Drawing for the job (mm, zero at the part's lowest x, y, z). Round coordinates to 2 decimals unless told otherwise and drop trailing zeros. Write each loop counter-clockwise with the first axis right and the second up, starting at its lowest first coordinate (ties: lowest second). Pieces come first, ordered by that corner, then holes.
Item 1: Band-saw the part on A-A, the plane x = 13.5. Write the cut outline in (y, z).
Item 2: Mould opens along Y. For the marked faces 1, 2, 3 and 4 say: +Y half, -Y half, draft (parallel to the pull), parting line (faces both ways), or undercut.
Item 3: Band-saw the part on D-D, the plane x = 25. Write the cut outline in (y, z), then the cut area to 4 significant figures.
Item 4: Wall check: probe 1 along Y at (x, z) = (13.5, 1.8); probe 2 along X at (y, z) = (14.5, 1.15). Give the ranges that are in metal, low to high.
Item 5: Band-saw the part on C-C, the plane z = 2.65. Count the separate pieces of the cut face and the enclosed holes in it, then the cut area to 3 significant figures.
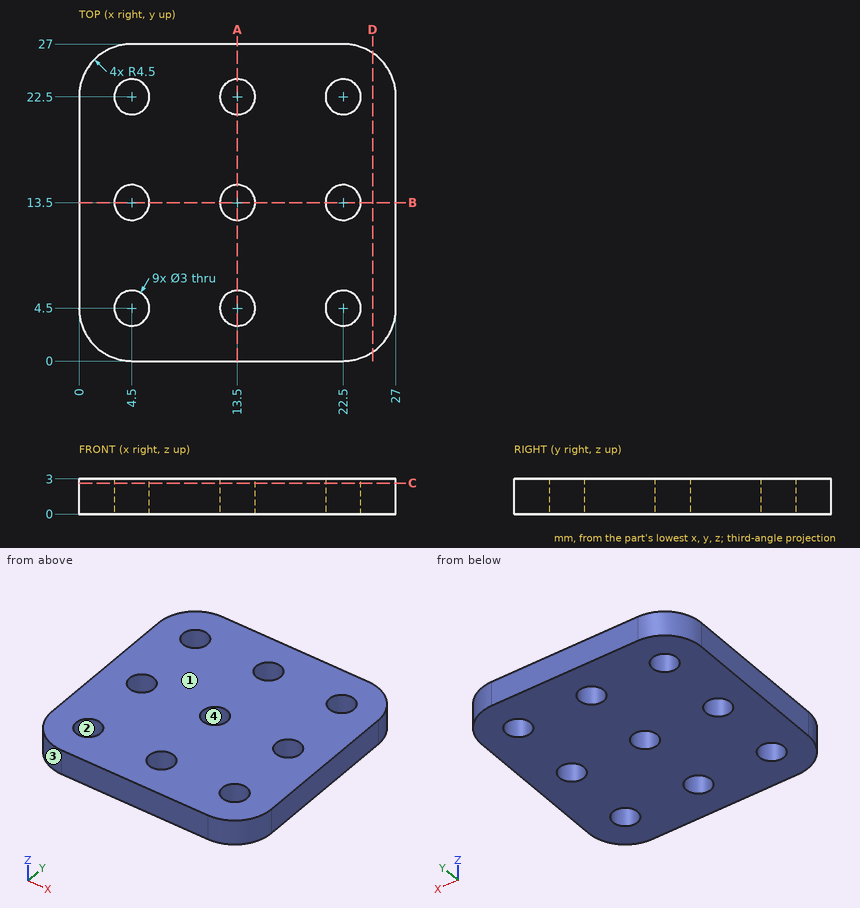
Results:
1. outline: (0, 0) - (3, 0) - (3, 3) - (0, 3) - close; (6, 0) - (12, 0) - (12, 3) - (6, 3) - close; (15, 0) - (21, 0) - (21, 3) - (15, 3) - close; (24, 0) - (27, 0) - (27, 3) - (24, 3) - close
2. face 1: draft
2. face 2: undercut
2. face 3: -Y half
2. face 4: undercut
3. outline: (0.76, 0) - (26.24, 0) - (26.24, 3) - (0.76, 3) - close
3. area: 76.45 mm2
4. probe 1: y = 0 to 3, 6 to 12, 15 to 21, 24 to 27
4. probe 2: x = 0 to 3.38, 5.62 to 12.38, 14.62 to 21.38, 23.62 to 27
5. separate pieces: 1
5. enclosed holes: 9
5. area: 648 mm2
